Input: dimensioned drawing with shaded views. Units: mm. Origin: part minimum x, y, z. A direction names the side the tool comes from. Give positions to 0.01 mm unless a question says otherwise; leave off trailing zeros. Write each loop counter-clockwise with the first axis right and the second up, starting at its lowest first coordinate (ties: lowest second). Pieces come first, ordered by that corner, then holes.
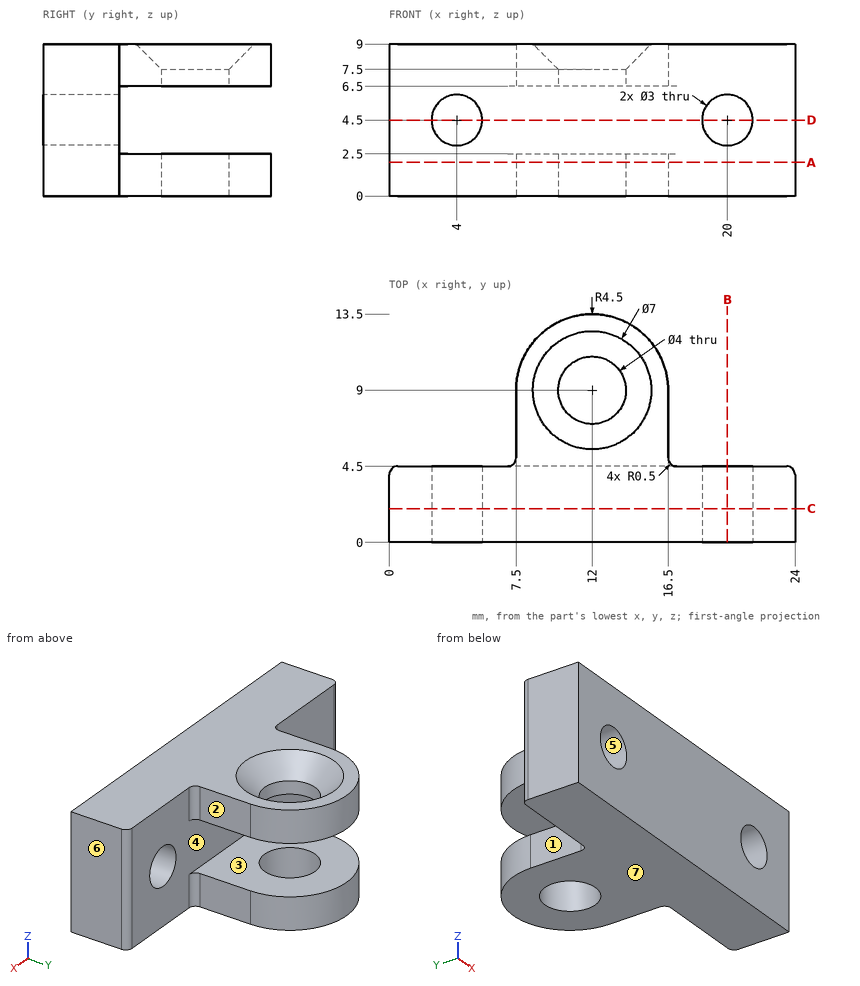
Item 1: Section C-C (y = 2). Return loops of the section in (x, z).
Item 2: Set-up query: the marked faces 1, 2, 3 and 4. Return all of +Z, -Z, +X, -X, +Y, -Y with unobstructed straight access to the full face (end or side cutting, diameter ignored); none if empty.
Item 3: Mould query, pull axis Z, two halves, no side actions, for the marked faces 5, 6 and 7. Classes: +Z half, -Z half, draft (parallel to the pull), parting line (faces both ways), or undercut.
Item 4: Section A-A (z = 2). Return loops of the section in (x, y).
Item 5: Pin query (flat end, axial travel): pin 1 (2.5 mm diameter, centred on x = 12, y = 9, fed in from +Z); pin 2 (3 mm diameter, centred on y = 10, z = 3.5, fed in from -X); pin 3 (3 mm diameter, centred on y = 7, z = 8, fed in from +X); pin 4 (5 mm diameter, centred on x = 20, z = 4.5, fed in from +Y). Return the tip coordinate at first contact, or that it passes through.
Item 6: Ray query, line 1 (X direction, y = 2.3, z = 4.5); line 2 (X direction, y = 9, z = 6.85); line 3 (X direction, y = 4, z = 5.5). Return the intervals inside material, ascending.
Item 7: Section D-D (z = 4.5). Return loops of the section in (x, y).
Item 8: Section B-B (x = 20). Return loops of the section in (y, z).
Solved:
1. outline: (0, 0) - (24, 0) - (24, 9) - (0, 9) - close; hole circle Ø3 at (4, 4.5); hole circle Ø3 at (20, 4.5)
2. face 1: +Z, -Z, -X, +Y
2. face 2: +Z, -Z, +X, +Y
2. face 3: +X, -X, +Y
2. face 4: +Y
3. face 5: undercut
3. face 6: draft
3. face 7: -Z half
4. outline: (0, 0) - (24, 0) - (24, 4) arc R0.5 ccw to (23.5, 4.5) - (17, 4.5) arc R0.5 cw to (16.5, 5) - (16.5, 9) arc R4.5 ccw to (7.5, 9) - (7.5, 5) arc R0.5 cw to (7, 4.5) - (0.5, 4.5) arc R0.5 ccw to (0, 4) - close; hole circle Ø4 at (12, 9)
5. pin 1: passes through
5. pin 2: stops at x = 7.5
5. pin 3: stops at x = 16.5
5. pin 4: stops at y = 4.5
6. line 1: x = 0 to 2.5, 5.5 to 18.5, 21.5 to 24
6. line 2: x = 7.5 to 10, 14 to 16.5
6. line 3: x = 0 to 2.88, 5.12 to 18.88, 21.12 to 24
7. outline: (0, 0) - (2.5, 0) - (2.5, 4.5) - (0.5, 4.5) arc R0.5 ccw to (0, 4) - close; (5.5, 0) - (18.5, 0) - (18.5, 4.5) - (5.5, 4.5) - close; (21.5, 0) - (24, 0) - (24, 4) arc R0.5 ccw to (23.5, 4.5) - (21.5, 4.5) - close
8. outline: (0, 0) - (4.5, 0) - (4.5, 3) - (0, 3) - close; (0, 6) - (4.5, 6) - (4.5, 9) - (0, 9) - close
